Job drawing, mm, ordinate dimensions from the low corner. One solid piece. A direction names the side the tool comes from. Give positions to 0.01 mm unless a question says otherwise; leave off trailing zeros. Write each loop counter-clockwise with the first axis right and the second up, starting at its lowest first coordinate (ties: lowest second). Pieces come first, ordered by that corner, then holes. Notation, with made-up numbers: (-34, 16) -> (-18, 16) arc R22 ccw to (-18, 27) -> close; hole circle Ø5 at (9.25, -11). An arc over 180 degrees is marked (long way). Put each result on its own line as item: value. Start each with the question number.
Item 1: Slice it at C-C, the plane x = 23.5. List the corners of the cut face in (y, z), plus the area to 3 significant figures.
Item 2: Slice it at A-A, the plane z = 6. List the corners of the cut face in (x, y).
Item 3: Tool access for the marked faces 1, 2 and 3: list every direction of +Z, -Z, +X, -X, +Y, -Y with a clear straight run to the whole face (end or side of a thin tool).
Item 4: Flat gauge pins, fed straight in: pin 1 Ø6 at (x, y) = (62.5, 2.5) entering from +Z; pin 2 Ø4 at (x, y) = (40.5, 2.5) entering from +Z; pin 3 Ø2 at (x, z) = (21, 1.5) entering from -Y. Where does each tip first touch, or does it go through?
Item 5: Slice it at D-D, the plane x = 12. List the corners of the cut face in (y, z).
Item 6: Drill centre lines: line 1 along Y through (x, z) = (71, 6); line 2 along X through (y, z) = (4.75, 11); line 3 along Z through (x, y) = (23, 8.25). Where is each one in solid material? Low to high.
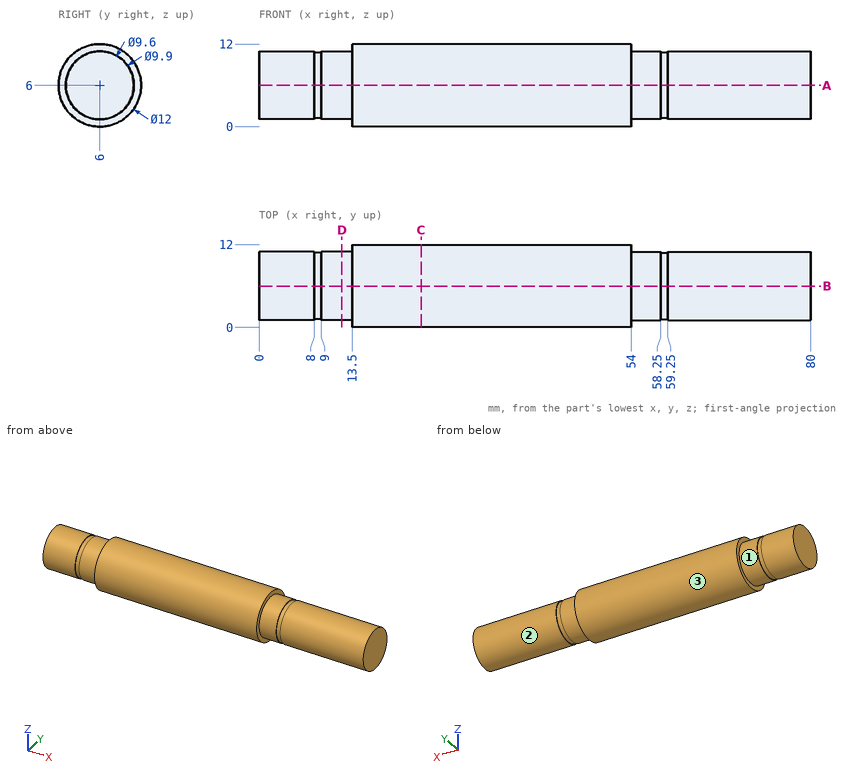
Values follow:
1. outline: circle Ø12 at (6, 6)
1. area: 113 mm2
2. outline: (0, 1.05) -> (8, 1.05) -> (8, 1.2) -> (9, 1.2) -> (9, 1.05) -> (13.5, 1.05) -> (13.5, 0) -> (54, 0) -> (54, 1.05) -> (58.25, 1.05) -> (58.25, 1.2) -> (59.25, 1.2) -> (59.25, 1.05) -> (80, 1.05) -> (80, 10.95) -> (59.25, 10.95) -> (59.25, 10.8) -> (58.25, 10.8) -> (58.25, 10.95) -> (54, 10.95) -> (54, 12) -> (13.5, 12) -> (13.5, 10.95) -> (9, 10.95) -> (9, 10.8) -> (8, 10.8) -> (8, 10.95) -> (0, 10.95) -> close
3. face 1: -X
3. face 2: +X
3. face 3: +X, -X
4. pin 1: z = 10.92
4. pin 2: z = 11.81
4. pin 3: y = 1.13
5. outline: circle Ø9.9 at (6, 6)
6. line 1: 1.05 to 10.95
6. line 2: 13.5 to 54
6. line 3: 0.44 to 11.56
